from build123d import *

# Parameters (mm, degrees)
F0_W     = 150
F0_H     = 140
F1_DEPTH = 47
F2_W     = 146
F2_H     = 136
F3_DEPTH = 45
F4_W     = 150
F4_H     = 140
F4_W_2   = 146
F4_H_2   = 136
F5_DEPTH = 3
F6_W     = 150
F6_H     = 140
F6_W_2   = 148
F6_H_2   = 138
F7_DEPTH = 3


with BuildPart() as f1:
    # F0 (on Top) → F1 (new body)
    with BuildSketch(Plane.XY):
        with Locations((77.499742, 70)):
            Rectangle(F0_W, F0_H)
    extrude(amount=F1_DEPTH)

    # F2 (on face) → F3 (cut)
    with BuildSketch(Plane.XY.offset(47)):
        with Locations((77.499742, 70)):
            Rectangle(F2_W, F2_H)
    extrude(amount=-F3_DEPTH, mode=Mode.SUBTRACT)

    # F4 (on face) → F5 (join)
    with BuildSketch(Plane.XY.offset(47)):
        with Locations((77.499742, 70)):
            Rectangle(F4_W, F4_H)
        with Locations((77.499742, 70)):
            Rectangle(F4_W_2, F4_H_2, mode=Mode.SUBTRACT)
    extrude(amount=F5_DEPTH)

    # F6 (on face) → F7 (cut)
    with BuildSketch(Plane.XY.offset(50)):
        with Locations((77.499742, 70)):
            Rectangle(F6_W, F6_H)
        with Locations((77.499742, 70)):
            Rectangle(F6_W_2, F6_H_2, mode=Mode.SUBTRACT)
    extrude(amount=-F7_DEPTH, mode=Mode.SUBTRACT)


solid = f1.part
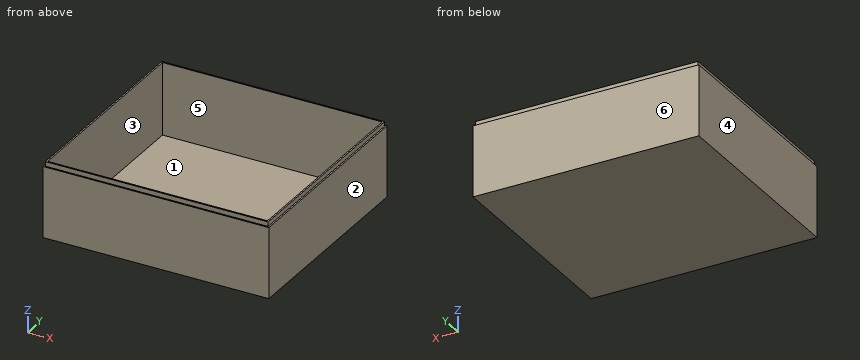
Input: part model. Units: mm. Frame: model coordinates. Face numbers are marked on the shaded views. A direction names the side the tool comes from. Coordinates: 2 decimals unless noted, no trailing zeros. Loops run counter-clockwise (first coordinate to the right, second up) from the corner with the lowest first, then second, coordinate; pieces in that order, holes last.
(1) Section B-B on x = 50. Return the cut outline in (y, z).
(2) Pull-direction query (X, two-part tool) for the marked faces 3, 4, 5 and 6; classes: released by +X, released by -X, zero draft, split by the parting line, or undercut.
(3) Set-up query: the marked faces 1 and 2. Return all of +Z, -Z, +X, -X, +Y, -Y with unobstructed straight access to the full face (end or side cutting, diameter ignored); none if empty.
(4) Section C-C on y = 123. Return the cut outline in (x, z), then the cut area to 3 significant figures.
(5) Section A-A on z = 15.5. Return the cut outline in (x, y).
(6) First-contact query: pin 1 Ø0.9 at (x, z) = (101, 48) entering from +Y; pin 2 Ø2 at (x, y) = (64, 67) entering from +Z; pin 3 Ø1.5 at (y, z) = (99.5, 48.5) entering from +X. Flat tips, straight axial feed; report the tip coordinate or a pass-through.
(7) Material intervals for probe 1 along Y at (x, z) = (141, 4); probe 2 along X at (y, z) = (122, 13.5); probe 3 along Z at (x, y) = (43.5, 67.5), sorted ascending.
Data:
1. outline: (0, 0) - (140, 0) - (140, 47) - (139, 47) - (139, 50) - (138, 50) - (138, 2) - (2, 2) - (2, 50) - (1, 50) - (1, 47) - (0, 47) - close
2. face 3: undercut
2. face 4: released by -X
2. face 5: undercut
2. face 6: zero draft
3. face 1: +Z
3. face 2: +Z, -Z, +X, +Y, -Y
4. outline: (2.5, 0) - (152.5, 0) - (152.5, 47) - (151.5, 47) - (151.5, 50) - (150.5, 50) - (150.5, 2) - (4.5, 2) - (4.5, 50) - (3.5, 50) - (3.5, 47) - (2.5, 47) - close
4. area: 486 mm2
5. outline: (2.5, 0) - (152.5, 0) - (152.5, 140) - (2.5, 140) - close; hole (4.5, 2) - (150.5, 2) - (150.5, 138) - (4.5, 138) - close
6. pin 1: stops at y = 139
6. pin 2: stops at z = 2
6. pin 3: stops at x = 151.5
7. probe 1: y = 0 to 2, 138 to 140
7. probe 2: x = 2.5 to 4.5, 150.5 to 152.5
7. probe 3: z = 0 to 2
